Can you work these out from the model? Positions are in its coordinate system, mm. A direction names the side the tool comes from. Round coordinates to 2 decimals unless told otherwise and drop trailing zeros. Loops run counter-clockwise (first coordinate to the right, second up) from the corner with the lowest first, then second, coordinate; pieces in that order, holes last. Notation, with made-up numbers: (3, 53) -> (53, 53) arc R18 cw to (53, 76) -> close; hole circle Ø1 at (-10, 20.25). An arc over 180 degrees is marked (long way). Write each question's results on one line, items separated by ' | '.
from build123d import *

# Parameters (mm, degrees)
BOSS_EXTRUDE1_DEPTH = 3.175
BOSS_EXTRUDE2_DEPTH = 25.4
SKETCH4_W           = 12.7
SKETCH4_H           = 3.175
BOSS_EXTRUDE3_DEPTH = 63.5


with BuildPart() as part:
    # Sketch1 → Boss-Extrude1 (new body)
    with BuildSketch(Plane.XY):
        Polygon((0, 101.6), (38.1, 101.6), (38.1, 76.2), (63.5, 76.2), (63.5, 0), (0, 0), align=None)
    extrude(amount=BOSS_EXTRUDE1_DEPTH)

    # Sketch2 → Boss-Extrude2 (add)
    with BuildSketch(Plane(origin=(63.5, 0, 0), x_dir=(0, 0, -1), z_dir=(1, 0, 0))):
        with BuildLine():
            Line((-3.175, 76.2), (0, 76.2))
            ThreePointArc((0, 76.2), (-3.62295396, 90.12573242), (-13.573125, 100.520246123))
            Line((-13.573125, 100.520246123), (-15.24, 97.817996554))
            ThreePointArc((-15.24, 97.817996554), (-6.39540352, 88.578428818), (-3.175, 76.2))
        make_face()
    extrude(amount=-BOSS_EXTRUDE2_DEPTH)

    # Sketch4 → Boss-Extrude3 (add)
    with BuildSketch(Plane(origin=(63.5, 0, 0), x_dir=(0, 0, -1), z_dir=(1, 0, 0))):
        with Locations((-6.35, 1.5875)):
            Rectangle(SKETCH4_W, SKETCH4_H)
    extrude(amount=-BOSS_EXTRUDE3_DEPTH)


solid = part.part
1. If we section it at C-C (x = 42.5): List the corners of the cut face in (y, z) for me (3 decimals), then the cut area to 3 significant figures.
Final values:
outline: (0, 0) -> (76.2, 0) arc R28.575 ccw to (100.52, 13.573) -> (97.818, 15.24) arc R25.4 cw to (76.2, 3.175) -> (3.175, 3.175) -> (3.175, 12.7) -> (0, 12.7) -> close | area: 359 mm2
2. If we section it at A-A (z = 10): List the corners of the cut face in (x, y) for me (3 decimals).
Final values:
outline: (0, 0) -> (63.5, 0) -> (63.5, 3.175) -> (0, 3.175) -> close; (38.1, 93.524) -> (63.5, 93.524) -> (63.5, 97.914) -> (38.1, 97.914) -> close
3. If we section it at D-D (y = 25): List the corners of the cut face in (x, z) for me (3 decimals).
Final values:
outline: (0, 0) -> (63.5, 0) -> (63.5, 3.175) -> (0, 3.175) -> close
4. On a 3-axis mill with a long thin cutter (end or side, diameter ignored), from which of +Z, -Z, +X, -X, +Y, -Y can I reach the whole of each face in a straight line? I mean faces 5 (the face through (38.1, 92, 2)), 6 (the face through (32, 2, 12.7)), 7 (the face through (38.1, 93, 8)), 8 (the face through (50.978, 88.736, 6.484)). Say none if no direction works.
Final values:
face 5: -Z, +X, +Y | face 6: +Z, +X, -X, -Y | face 7: +Z, -X, +Y | face 8: +Z, +X, -X
5. We'd pull the mould along Y, two halves only. Please class faces 1 (the face through (63.5, 50, 3)), 2 (the face through (32, 53, 3.175)), 3 (the face through (50.978, 99.188, 14.395)), 4 (the face through (32, 0, 6)): pulls with the +Y half, pulls with the -Y half, needs draft (parallel to the pull), parting line crosses it, or undercut.
Final values:
face 1: needs draft | face 2: undercut | face 3: pulls with the +Y half | face 4: pulls with the -Y half
6. If we section it at B-B (y = 92): List the corners of the cut face in (x, z) for me (3 decimals), then the cut area to 3 significant figures.
Final values:
outline: (0, 0) -> (38.1, 0) -> (38.1, 3.175) -> (0, 3.175) -> close; (38.1, 4.766) -> (63.5, 4.766) -> (63.5, 8.687) -> (38.1, 8.687) -> close | area: 221 mm2
7. Will these pins go through, and if not, where does the flat tip stop? pin 1 (2 mm diameter, centred on x = 49.5, z = 11.5, fed in from +Y); pin 2 (19 mm diameter, centred on x = 41, y = 77, fed in from +Z); pin 3 (1.6 mm diameter, centred on x = 32, y = 1, fed in from +Z).
Final values:
pin 1: y = 99.82 | pin 2: z = 5.36 | pin 3: z = 12.7
8. Please list where these lines run through material, in increasing order: line 1 (Y direction, x = 34, z = 4) (3 decimals); line 2 (Y direction, x = 47, z = 5.5) (3 decimals). Write a range as from..to.
Final values:
line 1: 0..3.175 | line 2: 0..3.175, 86.816..93.055
